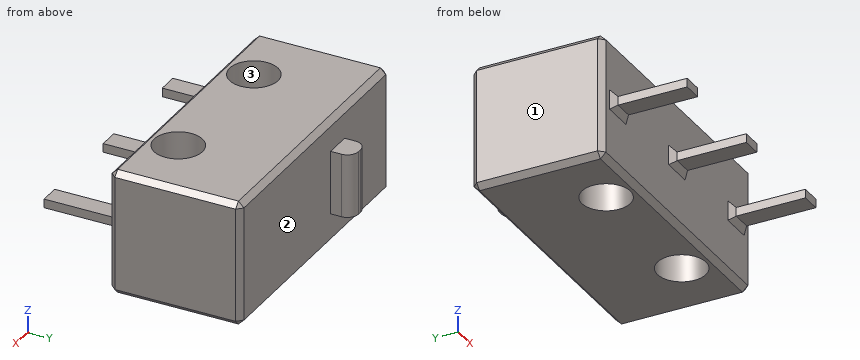
```python
from build123d import *

# Parameters (mm, degrees)
SCHIZZO1_W                   = 12.7
SCHIZZO1_H                   = 6
ESTRUSIONE_ESTRUSIONE1_DEPTH = 5.7
SCHIZZO2_W                   = 1.2
SCHIZZO2_H                   = 2.9
ESTRUSIONE_ESTRUSIONE2_DEPTH = 1
SCHIZZO3_R                   = 1.1
TAGLIO_ESTRUSIONE1_DEPTH     = 10.424038412
RACCORDO1_R                  = 0.5
SCHIZZO4_W                   = 0.9
SCHIZZO4_H                   = 0.4
ESTRUSIONE_ESTRUSIONE3_DEPTH = 3.4
RIPETIZIONE_A_L1_COUNT       = 2
RIPETIZIONE_A_L1_PITCH       = 5.08
RIPETIZIONE_A_L1_COL_COUNT   = 2
RIPETIZIONE_A_L1_COL_PITCH   = 5.08
SMUSSO1_SIZE                 = 0.25


with BuildPart() as part:
    # Schizzo1 → Estrusione-Estrusione1 (new body)
    with BuildSketch(Plane.XY):
        Rectangle(SCHIZZO1_W, SCHIZZO1_H)
    extrude(amount=ESTRUSIONE_ESTRUSIONE1_DEPTH)

    # Schizzo2 → Estrusione-Estrusione2 (add)
    with BuildSketch(Plane(origin=(0, 3, 0), x_dir=(1, 0, 0), z_dir=(0, 1, 0))):
        with Locations((-1.95, -2.85)):
            Rectangle(SCHIZZO2_W, SCHIZZO2_H)
    extrude(amount=ESTRUSIONE_ESTRUSIONE2_DEPTH)

    # Schizzo3 → Taglio-Estrusione1 (cut, through all)
    with BuildSketch(Plane.XY.offset(5.7)):
        with Locations((-3.25, -1.5)):
            Circle(SCHIZZO3_R)
        with Locations((3.25, -1.5)):
            Circle(SCHIZZO3_R)
    extrude(amount=-TAGLIO_ESTRUSIONE1_DEPTH, mode=Mode.SUBTRACT)

    # Raccordo1
    raccordo1_edges = [part.edges().sort_by_distance(p)[0] for p in [
        (-1.35, 4, 2.85),
        (-2.55, 4, 2.85),
    ]]
    fillet(raccordo1_edges, radius=RACCORDO1_R)

    # Schizzo4 → Estrusione-Estrusione3 (add)
    with BuildSketch(Plane.XZ.offset(3)):
        with Locations((0, 2.85)):
            Rectangle(SCHIZZO4_W, SCHIZZO4_H)
    estrusione_estrusione3 = extrude(amount=ESTRUSIONE_ESTRUSIONE3_DEPTH)

    # Ripetizione a L1: Estrusione-Estrusione3 ×2
    with Locations(*[(i * RIPETIZIONE_A_L1_PITCH, 0, 0) for i in range(1, RIPETIZIONE_A_L1_COUNT)]):
        add(estrusione_estrusione3)

    # Ripetizione a L1 col: Estrusione-Estrusione3 ×2
    with Locations(*[(-i * RIPETIZIONE_A_L1_COL_PITCH, 0, 0) for i in range(1, RIPETIZIONE_A_L1_COL_COUNT)]):
        add(estrusione_estrusione3)

    # Smusso1
    smusso1_edges = [part.edges().sort_by_distance(p)[0] for p in [
        (-6.35, 0, 5.7),
        (0, -3, 5.7),
        (6.35, 0, 5.7),
        (0, -3, 0),
        (0.45, -3, 2.85),
        (0, -3, 3.05),
        (-0.45, -3, 2.85),
        (0, -3, 2.65),
        (-6.35, 0, 0),
        (0, 3, 0),
        (6.35, 0, 0),
        (5.53, -3, 2.85),
        (5.08, -3, 3.05),
        (4.63, -3, 2.85),
        (5.08, -3, 2.65),
        (-4.63, -3, 2.85),
        (-5.08, -3, 3.05),
        (-5.53, -3, 2.85),
        (-5.08, -3, 2.65),
        (6.35, -3, 2.85),
        (-6.35, -3, 2.85),
        (-6.35, 3, 2.85),
        (6.35, 3, 2.85),
        (0, 3, 5.7),
    ]]
    chamfer(smusso1_edges, length=SMUSSO1_SIZE)


solid = part.part
```
The listing builds one solid part. Answer for the finished solid, in the listing's coordinates (mm). Face numbers are marked on the shaded views. Coordinates: 2 decimals unless noted, no trailing zeros. Order: outer loops, then holes, each group sorted by start corner. A loop starts at its lowest first (then second) coordinate and runs counter-clockwise, first axis right, second up. Notation, with made-up numbers: M 15.5,4 L 32.5,4 A14 ccw 32.5,13 Z; hole C 43,38 d8. An arc over 180 degrees is marked long. Answer as a JSON object with one key per item and string values. Group by question number.
1. Flat-ended cylindrical pins translate along their axes: P1, Ø1, axis at x = 5, z = 1.5, coming from the +Y side; P2, Ø3, axis at x = 0, z = 3.5, coming from the +Y side; P3, Ø0.5, axis at x = -5, y = -4, coming from the +Z side. Find the tip coordinate at first contact, or state that the pin passes through.
2. Section A-A on y = -1.5 is taken. Write down the section's boundary in (x, z).
3. Section B-B on x = 3.25 is taken. Write down the section's boundary in (y, z).
4. Determine the mould class of the marked faces 1, 2 and 3 for opening direction X: released by +X, released by -X, zero draft, split by the parting line, or undercut.
5. Section C-C on z = 0.65 is taken. Write down the section's boundary in (x, y).
6. Straight lines are drawn through the part: line 1 (X direction, y = -2.5, z = 1.85); line 2 (Y direction, x = -3.25, z = 1.35); line 3 (X direction, y = -2.25, z = 3.95). For each, find the intervals that lie inside material, in ascending order.
7. Section D-D on y = -4.5 is taken. Write down the section's boundary in (x, z), then the cut area to 3 significant figures.
Values follow:
{
 "1": {"P1": "y = 3", "P2": "y = 3.86", "P3": "z = 3.05"},
 "2": {"outline": "M -6.35,0.25 L -6.1,0 L -4.35,0 L -4.35,5.7 L -6.1,5.7 L -6.35,5.45 Z; M -2.15,0 L 2.15,0 L 2.15,5.7 L -2.15,5.7 Z; M 4.35,0 L 6.1,0 L 6.35,0.25 L 6.35,5.45 L 6.1,5.7 L 4.35,5.7 Z"},
 "3": {"outline": "M -3,0.25 L -2.75,0 L -2.6,0 L -2.6,5.7 L -2.75,5.7 L -3,5.45 Z; M -0.4,0 L 2.75,0 L 3,0.25 L 3,5.45 L 2.75,5.7 L -0.4,5.7 Z"},
 "4": {"face 1": "released by -X", "face 2": "zero draft", "face 3": "undercut"},
 "5": {"outline": "M -6.35,-2.75 L -6.1,-3 L 6.1,-3 L 6.35,-2.75 L 6.35,2.75 L 6.1,3 L -6.1,3 L -6.35,2.75 Z; hole C -3.25,-1.5 d2.2; hole C 3.25,-1.5 d2.2"},
 "6": {"line 1": "-6.35 to -3.71, -2.79 to 2.79, 3.71 to 6.35", "line 2": "-3 to -2.6, -0.4 to 3", "line 3": "-6.35 to -4.05, -2.45 to 2.45, 4.05 to 6.35"},
 "7": {"outline": "M -5.53,2.65 L -4.63,2.65 L -4.63,3.05 L -5.53,3.05 Z; M -0.45,2.65 L 0.45,2.65 L 0.45,3.05 L -0.45,3.05 Z; M 4.63,2.65 L 5.53,2.65 L 5.53,3.05 L 4.63,3.05 Z", "area": "1.08 mm2"}
}
